Verification items for this drawing (mm, ordinates from the low corner). Round coordinates to 2 decimals unless told otherwise and drop trailing zeros. Loops run counter-clockwise (first coordinate to the right, second up) from the corner with the lowest first, then second, coordinate; pieces in that order, holes last. Notation, with made-up numbers: M -14,-8 L -3,-8 A21 cw -3,12 Z; hole C 61,67 d5. An arc over 180 degrees is marked long. One line per item, written item: value.
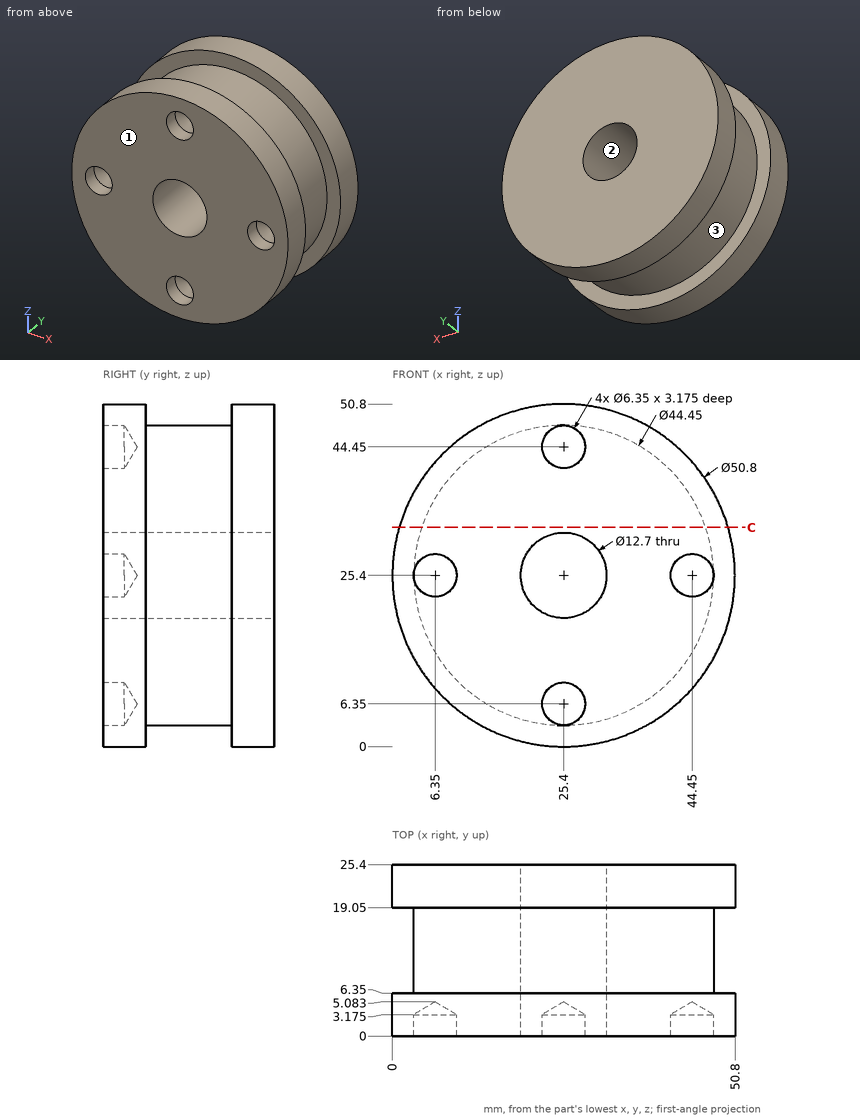
(1) Thickness scan on L1, parallel to Y at x = 35.5, z = 3; L2, parallel to Z at x = 27.5, y = 6; L3, parallel to X at y = 1.2, z = 6.35 (1 decimal). Record the ranges inside material, lowest first. Write a range as from..to.
Completed:
L1: y = 0..6.35, 19.05..25.4
L2: z = 0.09..19.41, 31.39..50.71
L3: x = 8.6..22.2, 28.6..42.2
(2) Sectioned sample at C-C on z = 32.5. Enter the section's corners in (x, y).
Completed:
outline: M 1.01,0 L 49.79,0 L 49.79,6.35 L 46.46,6.35 L 46.46,19.05 L 49.79,19.05 L 49.79,25.4 L 1.01,25.4 L 1.01,19.05 L 4.34,19.05 L 4.34,6.35 L 1.01,6.35 Z
(3) Depth check by flat-ended pin: pin 1 Ø7.5 at (x, z) = (44.45, 25.4) entering from -Y; pin 2 Ø12 at (y, z) = (21.5, 33.5) entering from -X; pin 3 Ø10 at (y, z) = (6.5, 12.5) entering from +X; pin 4 Ø3 at (x, y) = (20, 4.5) entering from +Z. Enter the tip coordinate at first touch or a pass-through.
Completed:
pin 1: stops at y = 0
pin 2: stops at x = 0.09
pin 3: stops at x = 49.54
pin 4: stops at z = 50.5
(4) Mould release check, pull along X, two halves, no side actions. Record for the marked faces 1, 2 and 3: +X half, -X half, draft (parallel to the pull), parting line (faces both ways), or undercut.
Completed:
face 1: draft
face 2: undercut
face 3: parting line
